Read the model definition and answer for the solid it produces. Units are mm, in the model's axes. Face numbers are marked on the shaded views. A direction names the side the tool comes from. Round coordinates to 2 decimals unless told otherwise and drop trailing zeros. Order: outer loops, then holes, each group sorted by start corner. A loop starts at its lowest first (then second) coordinate and runs counter-clockwise, first axis right, second up. Notation, with made-up numbers: (-19, -14.75) -> (23, -14.75) arc R15 cw to (23, 4.25) -> close; hole circle Ø8 at (80, 41). An arc over 180 degrees is marked (long way). Use a Markdown table: item, result. Add a question column.
1. Section C-C, the plane y = -9 is taken. Give the vertices of the cut face in (x, z).
2. Section A-A, the plane x = -12 is taken. Give the vertices of the cut face in (y, z).
3. For the marked faces 5 and 6, determine the directions among +Z, -Z, +X, -X, +Y, -Y from which every point of the face is accessible in a straight line to the end or side of a thin tool.
4. Consider L1, parallel to Y at x = 14, z = 40.5; L2, parallel to Z at x = -11, y = -8. Determine where each line is inside the solid, lowest interval first. Write a range as [from, to].
5. The mould has two halves that part along Z. Classify the marked faces 1, 2, 3 and 4: +Z half, -Z half, draft (parallel to the pull), parting line (faces both ways), or undercut.
6. Section B-B, the plane z = 48 is taken. Give the vertices of the cut face in (x, y), then the cut area to 3 significant figures.
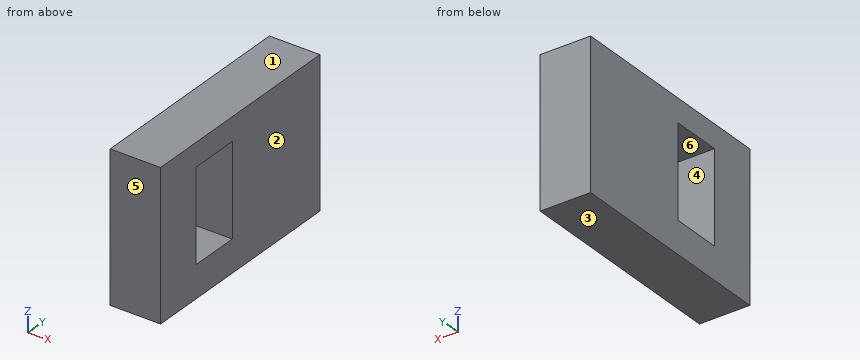
```python
from build123d import *

# Parameters (mm, degrees)
SKETCH2_W           = 146.376941915
SKETCH2_H           = 218.632716635
BOSS_EXTRUDE2_DEPTH = 25
CUT_EXTRUDE1_DEPTH  = 50


with BuildPart() as part:
    # Sketch2 → Boss-Extrude2 (new, symmetric)
    with BuildSketch(Plane(origin=(0, 0, 0), x_dir=(0, 0, -1), z_dir=(1, 0, 0))):
        with Locations((-3.490539111, 10.898614686)):
            Rectangle(SKETCH2_W, SKETCH2_H)
    extrude(amount=BOSS_EXTRUDE2_DEPTH, both=True)

    # Sketch1 → Cut-Extrude1 (cut)
    with BuildSketch(Plane(origin=(0, 0, 0), x_dir=(1, 0, 0), z_dir=(0, 1, 0))):
        with BuildLine():
            Line((28.234849526, 37.73567567), (-25.290931566, 37.73567567))
            add(Edge.make_bspline(
                [(-25.290931566, 37.73567567), (-30.76189097, 7.536622835), (-30.130821337, -23.0684525), (-31.981654202, -53.525781092)],
                knots=[0, 0, 0, 0, 1, 1, 1, 1], degree=3))
            Line((-31.981654202, -53.525781092), (35.996087784, -53.525781092))
            add(Edge.make_bspline(
                [(28.234849526, 37.73567567), (39.487990314, 7.96851172), (30.114114901, -23.184955899), (35.996087784, -53.525781092)],
                knots=[0, 0, 0, 0, 1, 1, 1, 1], degree=3))
        make_face()
    extrude(amount=-CUT_EXTRUDE1_DEPTH, mode=Mode.SUBTRACT)


solid = part.part
```
Verdict:
| question | item | result |
|---|---|---|
| 1 | outline | (-25, -69.7) -> (25, -69.7) -> (25, -37.74) -> (-25, -37.74) -> close; (-25, 53.53) -> (25, 53.53) -> (25, 76.68) -> (-25, 76.68) -> close |
| 2 | outline | (-98.42, -69.7) -> (120.21, -69.7) -> (120.21, 76.68) -> (-98.42, 76.68) -> close; hole (-50, -37.74) -> (0, -37.74) -> (0, 53.53) -> (-50, 53.53) -> close |
| 3 | face 5 | +Z, -Z, +X, -X, -Y |
| 3 | face 6 | +X, -X |
| 4 | L1 | y = [-98.42, -50], [0, 120.21] |
| 4 | L2 | z = [-69.7, -37.74], [53.53, 76.68] |
| 5 | face 1 | +Z half |
| 5 | face 2 | draft |
| 5 | face 3 | -Z half |
| 5 | face 4 | undercut |
| 6 | outline | (-25, -98.42) -> (25, -98.42) -> (25, -50) -> (-25, -50) -> close; (-25, 0) -> (25, 0) -> (25, 120.21) -> (-25, 120.21) -> close |
| 6 | area | 8,430 mm2 |
